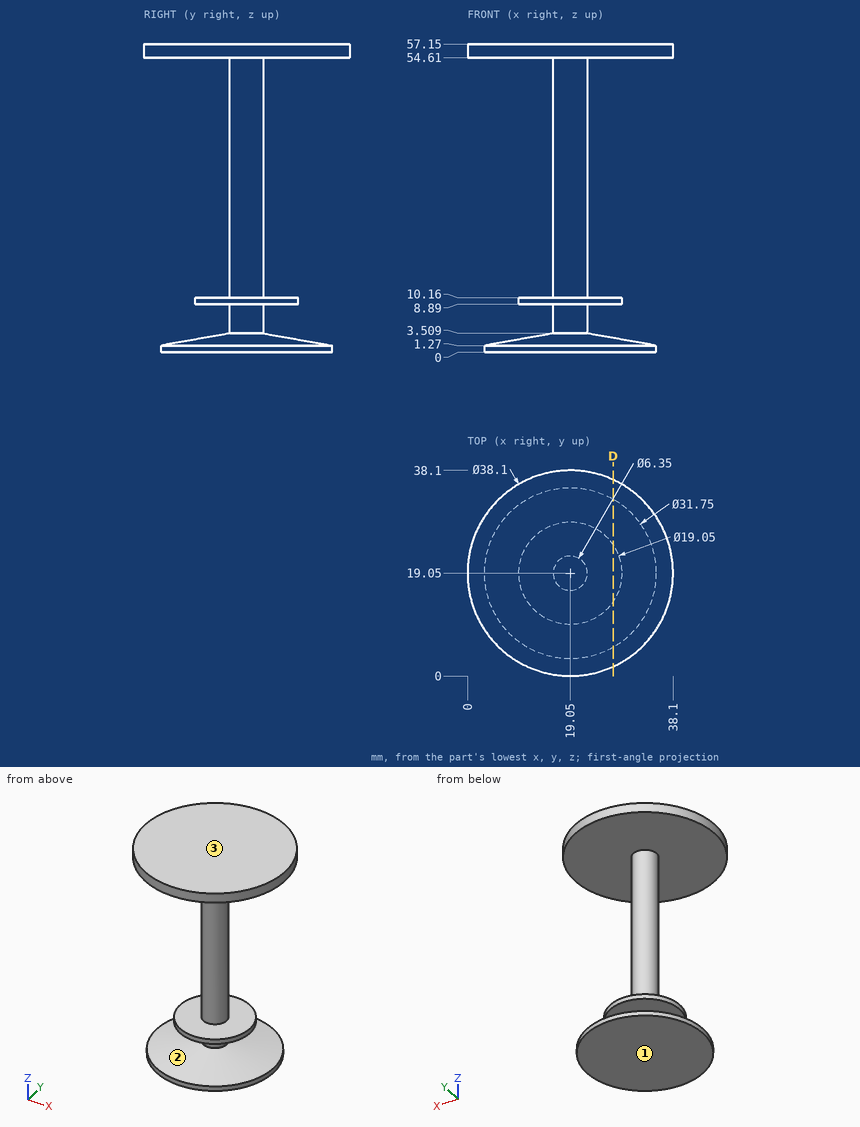
Input: dimensioned drawing with shaded views. Units: mm. Origin: part minimum x, y, z. Give positions to 0.01 mm unless a question says otherwise; leave off trailing zeros. Use a Markdown table: item, result.
1) Section query D-D, the plane x = 27. Count the separate pieces of the cut face and the enclosed holes in it, then the cut area to 3 significant figures.
Answer list:
| item | result |
|---|---|
| separate pieces | 3 |
| enclosed holes | 0 |
| area | 160 mm² |
2) Ray query, line 1 along Z through (x, y) = (9.5, 17); line 2 along Z through (x, y) = (20.5, 25.5); line 3 along Z through (x, y) = (14, 6). Return the intervals inside material, ascending. Write a range as [from, to].
Answer list:
| item | result |
|---|---|
| line 1 | [0, 2.35], [54.61, 57.15] |
| line 2 | [0, 2.9], [8.89, 10.16], [54.61, 57.15] |
| line 3 | [0, 1.6], [54.61, 57.15] |
3) Contact query for flat-ended pins moving along their axis: P1, Ø8, axis at y = 10, z = 9, coming from the -X side; P2, Ø1, axis at x = 21, z = 19, coming from the +Y side (1 decimal); P3, Ø10, axis at y = 20.5, z = 40.5, coming from the +X side (3 decimals). Output: stop coordinate, or through.
Answer list:
| item | result |
|---|---|
| P1 | x = 10.97 |
| P2 | y = 21.9 |
| P3 | x = 22.225 |
4) Mould query, pull axis Z, two halves, no side actions, for the marked faces 1, 2 and 3. Classes: +Z half, -Z half, draft (parallel to the pull), parting line (faces both ways), or undercut.
Answer list:
| item | result |
|---|---|
| face 1 | -Z half |
| face 2 | undercut |
| face 3 | +Z half |
